from build123d import *

# Parameters (mm, degrees)
SKETCH1_R           = 3.25
BOSS_EXTRUDE1_DEPTH = 2.5
SKETCH2_R           = 1.75
CUT_EXTRUDE1_DEPTH  = 2.5
SKETCH3_W           = 12.5
SKETCH3_H           = 7.2
BOSS_EXTRUDE2_DEPTH = 5
FILLET1_R           = 2.54
FILLET2_R           = 0.75


with BuildPart() as part:
    # Sketch1 → Boss-Extrude1 (new body)
    with BuildSketch(Plane(origin=(0, 0, 0), x_dir=(1, 0, 0), z_dir=(0, 1, 0))):
        Circle(SKETCH1_R)
    extrude(amount=BOSS_EXTRUDE1_DEPTH)

    # Sketch2 → Cut-Extrude1 (cut)
    with BuildSketch(Plane.XZ):
        Circle(SKETCH2_R)
    extrude(amount=-CUT_EXTRUDE1_DEPTH, mode=Mode.SUBTRACT)

    # Sketch3 → Boss-Extrude2 (add)
    with BuildSketch(Plane(origin=(0, 2.5, 0), x_dir=(1, 0, 0), z_dir=(0, 1, 0))):
        Rectangle(SKETCH3_W, SKETCH3_H)
    extrude(amount=BOSS_EXTRUDE2_DEPTH)

    # Fillet1
    fillet1_edges = [part.edges().sort_by_distance(p)[0] for p in [
        (6.25, 5, 3.6),
        (6.25, 5, -3.6),
        (-6.25, 5, -3.6),
        (-6.25, 5, 3.6),
    ]]
    fillet(fillet1_edges, radius=FILLET1_R)

    # Fillet2
    fillet2_edges = [part.edges().sort_by_distance(p)[0] for p in [
        (-6.25, 7.5, 0),
        (0, 7.5, -3.6),
        (6.25, 7.5, 0),
        (0, 7.5, 3.6),
        (-5.506051224, 7.5, 2.856051224),
        (5.506051224, 7.5, 2.856051224),
        (5.506051224, 7.5, -2.856051224),
        (-5.506051224, 7.5, -2.856051224),
    ]]
    fillet(fillet2_edges, radius=FILLET2_R)


solid = part.part
Geometry check sheet. Reference: the model listing, model coordinates, mm. A direction names the side the tool comes from. Coordinates: 2 decimals unless noted, no trailing zeros. Order: outer loops, then holes, each group sorted by start corner. A loop starts at its lowest first (then second) coordinate and runs counter-clockwise, first axis right, second up. Notation, with made-up numbers: (40, 27) -> (75, 27) arc R27 ccw to (75, 47) -> close; hole circle Ø10 at (56, 70). An arc over 180 degrees is marked (long way). Use a Markdown table: item, result. Add a question column.
1. Go/stop test with a flat-tipped pin: pin 1 Ø2 at (y, z) = (2.5, 2) entering from -X. Record where the tip stops, or that it passes through.
2. Material ranges on L1, parallel to Z at x = 0, y = 0.75; L2, parallel to Y at x = -3.5, z = 2.5; L3, parallel to X at y = 1.75, z = 0.5, recorded low to high.
3. Mould release check, pull along X, two halves, no side actions. Record for faces 1 (the face through (5.486, 4.655, 2.876)), 2 (the face through (1.617, 1.232, -0.67)), 3 (the face through (0, 7.5, 0)): pulls with the +X half, pulls with the -X half, needs draft (parallel to the pull), parting line crosses it, or undercut.
4. Set-up check for faces 4 (the face through (6.25, 5, 0)), 5 (the face through (0, 2.5, 0)): record each of +Z, -Z, +X, -X, +Y, -Y from which the full face is reachable in a straight line by a thin tool's end or side.
5. Cross-section at B-B (x = 0). Enter the section's corners in (y, z).
6. Cross-section at C-C (z = -0.5). Enter the section's corners in (x, y).
7. Cross-section at D-D (x = 2). Enter the section's corners in (y, z).
8. Cross-section at A-A (y = 6.5). Enter the section's corners in (x, z), and give its area (3 significant figures).
Filled sheet:
| question | item | result |
|---|---|---|
| 1 | pin 1 | x = -6.25 |
| 2 | L1 | -3.25 to -1.75, 1.75 to 3.25 |
| 2 | L2 | 2.5 to 7.5 |
| 2 | L3 | -3.21 to -1.68, 1.68 to 3.21 |
| 3 | face 1 | pulls with the +X half |
| 3 | face 2 | undercut |
| 3 | face 3 | needs draft |
| 4 | face 4 | +Z, -Z, +X, +Y, -Y |
| 4 | face 5 | -Y |
| 5 | outline | (0, -3.25) -> (2.5, -3.25) -> (2.5, -3.6) -> (6.75, -3.6) arc R0.75 ccw to (7.5, -2.85) -> (7.5, 2.85) arc R0.75 ccw to (6.75, 3.6) -> (2.5, 3.6) -> (2.5, 3.25) -> (0, 3.25) -> (0, 1.75) -> (2.5, 1.75) -> (2.5, -1.75) -> (0, -1.75) -> close |
| 6 | outline | (-6.25, 2.5) -> (-3.21, 2.5) -> (-3.21, 0) -> (-1.68, 0) -> (-1.68, 2.5) -> (1.68, 2.5) -> (1.68, 0) -> (3.21, 0) -> (3.21, 2.5) -> (6.25, 2.5) -> (6.25, 6.75) arc R0.75 ccw to (5.5, 7.5) -> (-5.5, 7.5) arc R0.75 ccw to (-6.25, 6.75) -> close |
| 7 | outline | (0, -2.56) -> (2.5, -2.56) -> (2.5, -3.6) -> (6.75, -3.6) arc R0.75 ccw to (7.5, -2.85) -> (7.5, 2.85) arc R0.75 ccw to (6.75, 3.6) -> (2.5, 3.6) -> (2.5, 2.56) -> (0, 2.56) -> close |
| 8 | outline | (-6.25, -1.06) arc R2.54 ccw to (-3.71, -3.6) -> (3.71, -3.6) arc R2.54 ccw to (6.25, -1.06) -> (6.25, 1.06) arc R2.54 ccw to (3.71, 3.6) -> (-3.71, 3.6) arc R2.54 ccw to (-6.25, 1.06) -> close |
| 8 | area | 84.5 mm2 |
